Input: dimensioned drawing with shaded views. Units: mm. Origin: part minimum x, y, z. A direction names the side the tool comes from. Give positions to 0.01 mm unless a question says otherwise; leave off trailing zeros. Order: outer loops, then holes, each group sorted by start corner. A loop starts at its lowest first (then second) coordinate and runs counter-clockwise, first axis right, second up.
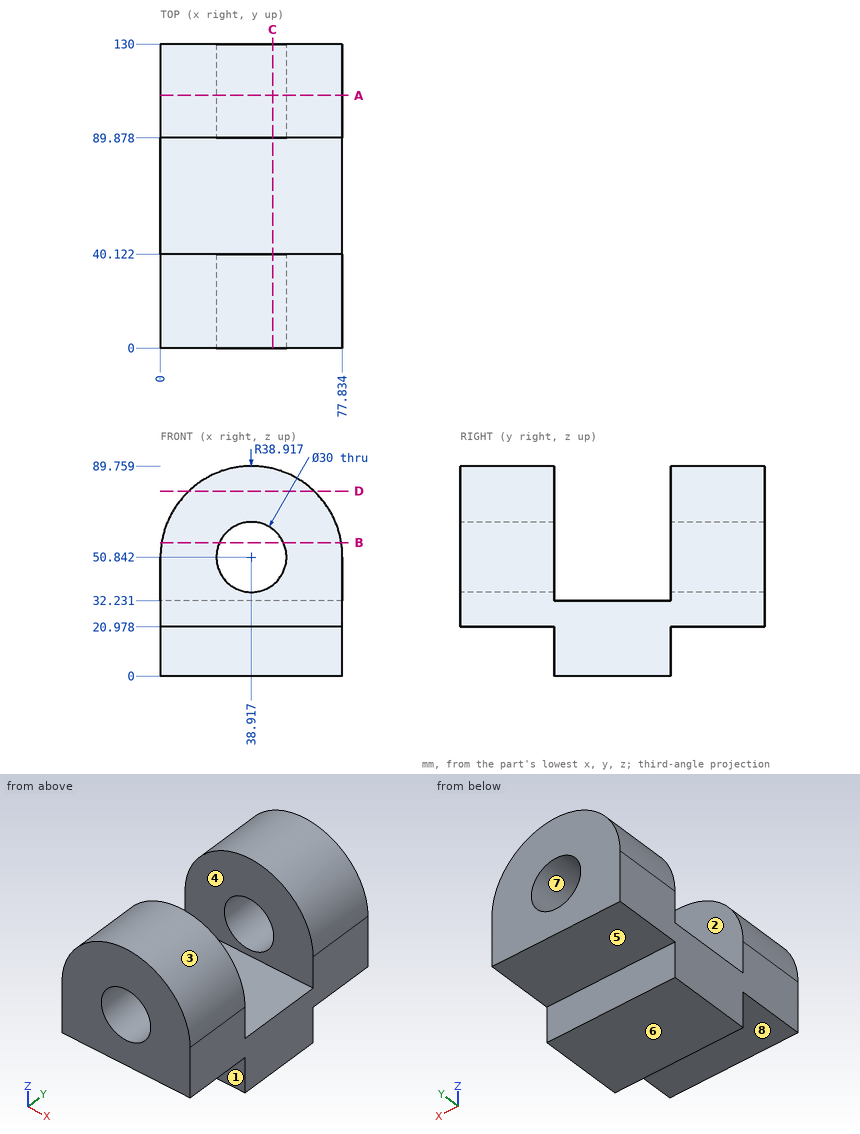
1) Material intervals for L1, parallel to Y at x = 55, z = 74; L2, parallel to Z at x = 29, y = 44.5; L3, parallel to Z at x = 41, y = 11.5, sorted ascending.
Report:
L1: y = 0 to 40.12, 89.88 to 130
L2: z = 0 to 32.23
L3: z = 20.98 to 35.99, 65.7 to 89.7
2) Reachability of the marked faces 4, 5, 6, 7 and 8 from +Z, -Z, +X, -X, +Y, -Y: full face, straight path, thin tool, end or side. Return the list, or none.
Report:
face 4: +Z, +X, -X
face 5: -Z, +X, -X, +Y
face 6: -Z, +X, -X, +Y, -Y
face 7: +Y, -Y
face 8: -Z, +X, -X, -Y
3) Draft query along Y for the marked faces 1, 2 and 3. Return one class per face: +Y half, -Y half, draft (parallel to the pull), parting line (faces both ways), or undercut.
Report:
face 1: -Y half
face 2: undercut
face 3: draft
4) Section query A-A, the plane y = 108. Return the cut outline in (x, z) (1 decimal).
Report:
outline: (0, 21) - (77.8, 21) - (77.8, 50.8) arc R38.9 ccw to (0, 50.8) - close; hole circle Ø30 at (38.9, 50.8)
5) Section query B-B, the plane z = 57. Return the cut outline in (x, y) (1 decimal), and give its area (3 significant figures).
Report:
outline: (0.5, 0) - (25.2, 0) - (25.2, 40.1) - (0.5, 40.1) - close; (0.5, 89.9) - (25.2, 89.9) - (25.2, 130) - (0.5, 130) - close; (52.6, 0) - (77.3, 0) - (77.3, 40.1) - (52.6, 40.1) - close; (52.6, 89.9) - (77.3, 89.9) - (77.3, 130) - (52.6, 130) - close
area: 3,970 mm2
6) Section query D-D, the plane z = 79. Return the cut outline in (x, y), and give its area (3 significant figures).
Report:
outline: (12.05, 0) - (65.78, 0) - (65.78, 40.12) - (12.05, 40.12) - close; (12.05, 89.88) - (65.78, 89.88) - (65.78, 130) - (12.05, 130) - close
area: 4,310 mm2
7) Pin query (flat end, axial travel): pin 1 (1 mm diameter, centred on y = 94, z = 54, fed in from -X); pin 2 (6.5 mm diameter, centred on x = 47.5, z = 7.5, fed in from +Y); pin 3 (3 mm diameter, centred on x = 27, z = 55.5, fed in from +Y); pin 4 (12 mm diameter, centred on x = 63, z = 77, fed in from -Y). Return the tip coordinate at first contact, or that it passes through.
Report:
pin 1: stops at x = 0.09
pin 2: stops at y = 89.88
pin 3: passes through
pin 4: stops at y = 0
8) Section query C-C, the plane x = 48. Return the cut outline in (y, z) (1 decimal).
Report:
outline: (0, 21) - (40.1, 21) - (40.1, 0) - (89.9, 0) - (89.9, 21) - (130, 21) - (130, 38.9) - (89.9, 38.9) - (89.9, 32.2) - (40.1, 32.2) - (40.1, 38.9) - (0, 38.9) - close; (0, 62.8) - (40.1, 62.8) - (40.1, 88.7) - (0, 88.7) - close; (89.9, 62.8) - (130, 62.8) - (130, 88.7) - (89.9, 88.7) - close
